Source: CAD feature listing. Evaluate the final solid. Frame: model axes, mm. Face numbers are marked on the shaded views. A direction names the side the tool comes from. Coordinates: 2 decimals unless noted, no trailing zeros. Write each loop counter-clockwise with the first axis right and the second up, starting at its lowest first coordinate (ties: lowest second). Pieces come first, ordered by that corner, then holes. Notation, with made-up numbers: M -14,3.5 L 6,3.5 A36 cw 6,42.5 Z; hole C 27.5,27 d3. An arc over 180 degrees is marked long. Write item = value, one per line. Start each with the question number.
1. Access query for the marked faces 1 and 2. Directions: +Z, -Z, +X, -X, +Y, -Y. A direction counts if a zero-diameter tool reaches every point of the face in a straight line with its end or side. Return the directions, or none.
2. Section query A-A (x = -7). Output: boundary loops of the cut face in (y, z).
3. Line query: line 1 along X through (y, z) = (24.8, 7); line 2 along X through (y, z) = (-14.5, 1); line 3 along Y through (x, z) = (-0.5, 7.25). Output: solid intervals per line, ascending.
4. Section query B-B (z = 7). Output: boundary loops of the cut face in (x, y).
5. Section query C-C (x = -1.25). Output: boundary loops of the cut face in (y, z), then the cut area to 3 significant figures.
6. Section query D-D (z = -4.75). Output: boundary loops of the cut face in (x, y), then the cut area to 3 significant figures.
7. Pin query (flat end, axial travel): pin 1 Ø2 at (x, z) = (-6, 7.5) entering from -Y; pin 2 Ø10 at (y, z) = (-10.5, -1) entering from -X. Return the tip coordinate at first contact, or that it passes through.
```python
from build123d import *

# Parameters (mm, degrees)
SKETCH1_W           = 20
SKETCH1_H           = 53
BOSS_EXTRUDE1_DEPTH = 3
SKETCH2_W           = 6
SKETCH2_H           = 3
BOSS_EXTRUDE2_DEPTH = 10
CUT_EXTRUDE1_REACH  = 53.962
SKETCH4_R           = 1.65


with BuildPart() as part:
    # Sketch1 → Boss-Extrude1 (new body)
    with BuildSketch(Plane(origin=(0, 0, 0), x_dir=(0, 0, -1), z_dir=(1, 0, 0))):
        Rectangle(SKETCH1_W, SKETCH1_H)
    extrude(amount=BOSS_EXTRUDE1_DEPTH)

    # Sketch2 → Boss-Extrude2 (add)
    with BuildSketch(Plane.ZY):
        with Locations((-7, 25)):
            Rectangle(SKETCH2_W, SKETCH2_H)
        with Locations((7, 25)):
            Rectangle(SKETCH2_W, SKETCH2_H)
    extrude(amount=BOSS_EXTRUDE2_DEPTH)

    # Sketch4 → Cut-Extrude1 (cut, up to next)
    with BuildSketch(Plane.XZ.offset(-23.5), mode=Mode.PRIVATE) as cut_extrude1_sk1:
        with Locations(Location((-7, 7, 0), (0, 0, 270))):
            Circle(SKETCH4_R)
    cut_extrude1_tool1 = extrude(cut_extrude1_sk1.sketch, amount=-CUT_EXTRUDE1_REACH, mode=Mode.PRIVATE) & part.part
    # Sketch4 → Cut-Extrude1 (cut, up to next)
    with BuildSketch(Plane.XZ.offset(-23.5), mode=Mode.PRIVATE) as cut_extrude1_sk2:
        with Locations(Location((-7, -7, 0), (0, 0, 270))):
            Circle(SKETCH4_R)
    cut_extrude1_tool2 = extrude(cut_extrude1_sk2.sketch, amount=-CUT_EXTRUDE1_REACH, mode=Mode.PRIVATE) & part.part
    add(cut_extrude1_tool1.solids().sort_by_distance((-7, 23.5, 7))[0], mode=Mode.SUBTRACT)
    add(cut_extrude1_tool2.solids().sort_by_distance((-7, 23.5, -7))[0], mode=Mode.SUBTRACT)


solid = part.part
```
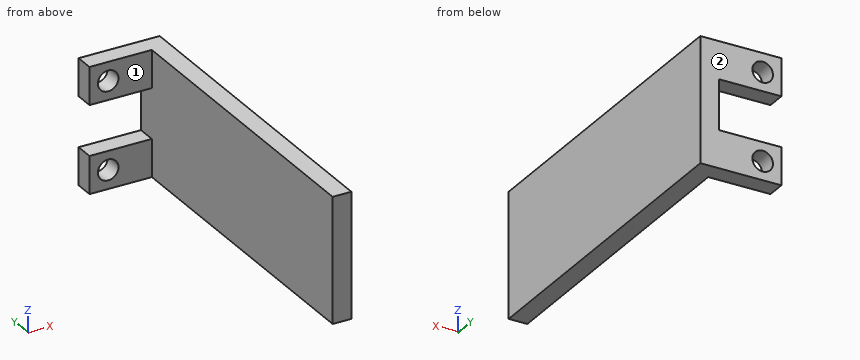
Results are:
q1.face_1 = +Z, -Z, -X, -Y
q1.face_2 = +Z, -Z, +X, -X, +Y
q2.outline = M 23.5,-10 L 26.5,-10 L 26.5,-8.65 L 23.5,-8.65 Z; M 23.5,-5.35 L 26.5,-5.35 L 26.5,-4 L 23.5,-4 Z; M 23.5,4 L 26.5,4 L 26.5,5.35 L 23.5,5.35 Z; M 23.5,8.65 L 26.5,8.65 L 26.5,10 L 23.5,10 Z
q3.line_1 = -10 to -8.65, -5.35 to 3
q3.line_2 = 0 to 3
q3.line_3 = 23.5 to 26.5
q4.outline = M -10,23.5 L -8.65,23.5 L -8.65,26.5 L -10,26.5 Z; M -5.35,23.5 L 0,23.5 L 0,-26.5 L 3,-26.5 L 3,26.5 L -5.35,26.5 Z
q5.outline = M 23.5,-10 L 26.5,-10 L 26.5,-4 L 23.5,-4 Z; M 23.5,4 L 26.5,4 L 26.5,10 L 23.5,10 Z
q5.area = 36.0 mm^2
q6.outline = M -10,23.5 L 0,23.5 L 0,-26.5 L 3,-26.5 L 3,26.5 L -10,26.5 Z
q6.area = 189 mm^2
q7.pin_1 = 23.5
q7.pin_2 = 0
